Input: dimensioned drawing with shaded views. Units: mm. Origin: part minimum x, y, z. Round coordinates to 2 decimals unless told otherwise and drop trailing zeros. Write each loop counter-clockwise with the first axis right and the second up, starting at its lowest first coordinate (ties: lowest second). Pieces come first, ordered by that corner, then holes. Notation, with made-up numbers: M -9,6.25 L 33,6.25 A32 cw 33,37.25 Z; hole C -37,47 d5. An arc over 180 degrees is marked long. Answer in a Markdown table with one row per item. Add a question column.
Item 1: Contact query for flat-ended pins moving along their axis: pin 1 (2 mm diameter, centred on x = 5, y = 27.5, fed in from +Z); pin 2 (1 mm diameter, centred on x = 5, y = 105, fed in from +Z); pin 3 (1 mm diameter, centred on x = 3, y = 34.5, fed in from +Z). Output: stop coordinate, or through.
Item 2: Cut plane C-C on x = 5. Return loops of the section in (y, z) (1 decimal).
Item 3: Cut plane D-D on y = 78. Return loops of the section in (x, z).
Item 4: Material intervals for probe 1 along Z at (x, y) = (2.5, 101.6); probe 2 along Z at (x, y) = (1.5, 145); probe 3 along Z at (x, y) = (5.75, 17.5) (1 decimal), sorted ascending.
Item 5: Cut plane A-A on z = 63.5. Return loops of the section in (x, y).
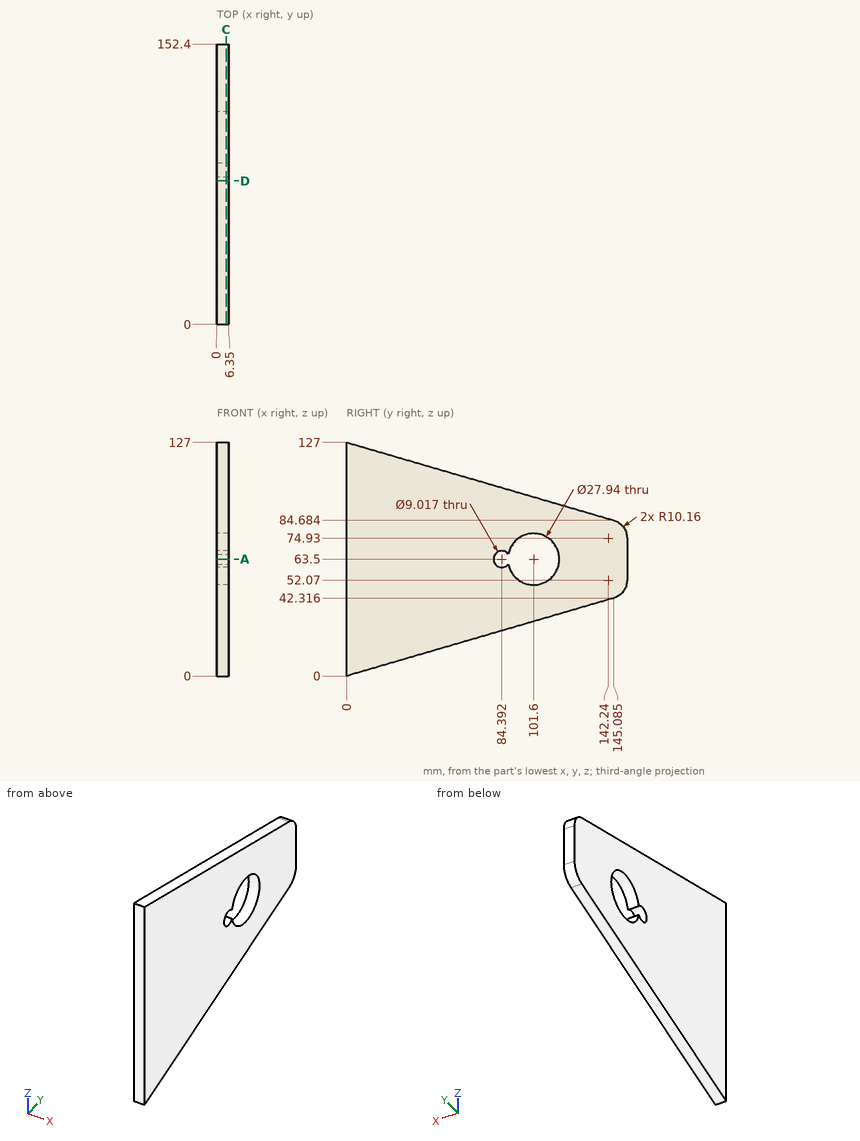
Results below:
| question | item | result |
|---|---|---|
| 1 | pin 1 | z = 119.27 |
| 1 | pin 2 | z = 96.52 |
| 1 | pin 3 | z = 117.08 |
| 2 | outline | M 0,0 L 145.1,42.3 A10.2 ccw 152.4,52.1 L 152.4,74.9 A10.2 ccw 145.1,84.7 L 0,127 Z; hole M 87.9,60.7 A14 ccw long 87.9,66.3 A4.5 ccw long Z |
| 3 | outline | M 0,22.75 L 6.35,22.75 L 6.35,104.25 L 0,104.25 Z |
| 4 | probe 1 | 29.63 to 49.53, 77.47 to 97.37 |
| 4 | probe 2 | 42.29 to 84.71 |
| 4 | probe 3 | 5.1 to 121.9 |
| 5 | outline | M 0,0 L 6.35,0 L 6.35,79.88 L 0,79.88 Z; M 0,115.57 L 6.35,115.57 L 6.35,152.4 L 0,152.4 Z |
